```python
from build123d import *

# Parameters (mm, degrees)
F1_DEPTH    = 40
F2_W        = 150
F2_H        = 2.5
F3_DEPTH    = 10
F4_T1_DEPTH = 175.7168298797
F5_R        = 5


# Not quite as in the source:
# - a fillet or chamfer that OpenCascade refuses, or shapes differently, is made with other operations: its cross-section is extruded or revolved along the edge and cut away or added


with BuildPart() as f1:
    # F0 (on Front) → F1 (new body)
    with BuildSketch(Plane.XZ):
        Polygon((150, 0), (0, 0), (0, -154.3005230276), (35, -154.3005230276), (45, -40), (105, -40), (115, -154.3005230276), (150, -154.3005230276), align=None)
    extrude(amount=F1_DEPTH)

    # F2 (on face) → F3 (cut)
    with BuildSketch(Plane.XZ.offset(40)):
        with Locations((75, -4.8898250982)):
            Rectangle(F2_W, F2_H)
    extrude(amount=-F3_DEPTH, mode=Mode.SUBTRACT)

    # F4: chamfer of 5 on 1 edges, made by hand

    # F4_s2 → F4_t1 (cut)
    with BuildSketch(Plane.YZ.offset(-12.8584149398)):
        Polygon((-35, 0), (-40, -5), (-40, 0), align=None)
    extrude(amount=F4_T1_DEPTH, mode=Mode.SUBTRACT)

    # F5
    f5_edges = [f1.edges().sort_by_distance(p)[0] for p in [
        (75, -35, 0),
    ]]
    fillet(f5_edges, radius=F5_R)


solid = f1.part
```
The listing builds one solid part. Answer for the finished solid, in the listing's coordinates (mm). A direction names the side the tool comes from. Give positions to 0.01 mm unless a question says otherwise; leave off trailing zeros. Write each loop counter-clockwise with the first axis right and the second up, starting at its lowest first coordinate (ties: lowest second). Pieces come first, ordered by that corner, then holes. Notation, with made-up numbers: (63, -28) - (77, -28) arc R22 cw to (77, 7) - close; hole circle Ø7 at (27.5, -26). An arc over 180 degrees is marked (long way). Use one line per item in the form item = value. Start each with the question number.
1) Consider line 1 along Z through (x, y) = (103.5, -31); line 2 along Z through (x, y) = (50, -17.5); line 3 along X through (y, z) = (-13.5, -56). Determine where each line is inside the solid, lowest interval first. Write a range as from..to.
2) Find section B-B on x = 84. Determine the outline of the cut face in (y, z).
3) A tool of negligible diameter and unlimited length cuts with its end or side. For faces 4 (the face through (75, -20, -40)), 5 (the face through (17, -20, -154.301)), 6 (the face through (74, -34, -3.64)), from which of +Z, -Z, +X, -X, +Y, -Y can it reach the whole face along a straight path? Write none if from no direction.
4) Find section D-D on x = 40. Determine the outline of the cut face in (y, z).
5) Flat-ended cylindrical pins translate along their axes: pin 1 Ø1.2 at (x, z) = (49, -4.5) entering from -Y; pin 2 Ø10 at (x, y) = (77.5, -31) entering from -Z; pin 3 Ø3 at (x, y) = (38, -36.5) entering from +Z. Find the tip coordinate at first contact, or state that the pin passes through.
6) Find section A-A on z = -105.5. Determine the outline of the cut face in (x, y).
7) The mould has two halves that part along X. Classify faces 1 (the face through (0, -20, -76)), 2 (the face through (109.93, -19.72, -96.35)), 3 (the face through (74, -35, -6.14)): pulls with the +X half, pulls with the -X half, needs draft (parallel to the pull), parting line crosses it, or undercut.
8) Find section C-C on y = -23. Determine the outline of the cut face in (x, z).
Geometry results:
q1.line_1 = -40..-6.14, -3.64..0
q1.line_2 = -40..0
q1.line_3 = 0..43.6, 106.4..150
q2.outline = (-40, -40) - (0, -40) - (0, 0) - (-32.93, 0) arc R5 ccw to (-36.46, -1.46) - (-38.64, -3.64) - (-30, -3.64) - (-30, -6.14) - (-40, -6.14) - close
q3.face_4 = -Z, +Y, -Y
q3.face_5 = -Z, +X, -X, +Y, -Y
q3.face_6 = +X, -X, -Y
q4.outline = (-40, -97.15) - (0, -97.15) - (0, 0) - (-32.93, 0) arc R5 ccw to (-36.46, -1.46) - (-38.64, -3.64) - (-30, -3.64) - (-30, -6.14) - (-40, -6.14) - close
q5.pin_1 = -30
q5.pin_2 = -40
q5.pin_3 = -0.45
q6.outline = (0, -40) - (39.27, -40) - (39.27, 0) - (0, 0) - close; (110.73, -40) - (150, -40) - (150, 0) - (110.73, 0) - close
q7.face_1 = pulls with the -X half
q7.face_2 = undercut
q7.face_3 = needs draft
q8.outline = (0, -154.3) - (35, -154.3) - (45, -40) - (105, -40) - (115, -154.3) - (150, -154.3) - (150, 0) - (0, 0) - close
